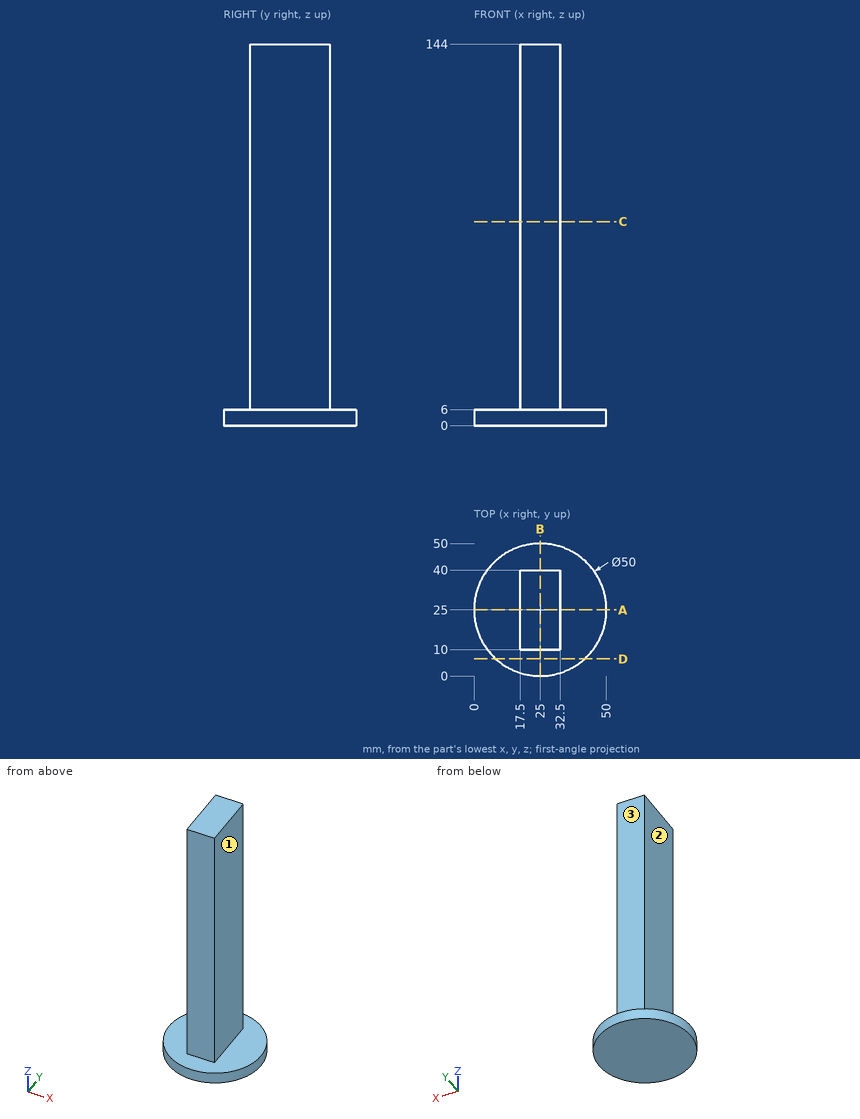
Print and shaded views of the part. All mm, measured from the part's lowest x, y and z. A direction names the side the tool comes from. Round coordinates to 2 decimals unless told otherwise and drop trailing zeros. Write each loop counter-clockwise with the first axis right and the second up, starting at its lowest first coordinate (ties: lowest second). Pieces come first, ordered by that corner, then holes.
(1) Slice it at C-C, the plane z = 77. Write the cut outline in (x, y).
(2) Slice it at D-D, the plane y = 6.5. Write the cut outline in (x, z).
(3) 3-axis set-ups, long thin cutter, end or side, ignore diameter. For the marked faces 1, 2 and 3: which of +Z, -Z, +X, -X, +Y, -Y reach the whole face in a straight line?
(4) Drop flat-ended pins along their axis: P1, Ø8, axis at x = 28.5, y = 23.5, coming from the -Z side; P2, Ø12, axis at x = 13, z = 18, coming from the -Y side; P3, Ø9, axis at y = 29, z = 60.5, coming from the -X side; P4, Ø24, axis at y = 29, z = 66.5, coming from the +X side. Give the stop position or say it passes through.
(5) Probe line 1 along Z through (x, y) = (34.5, 35); line 2 along Y through (x, z) = (21.5, 106); line 3 along X through (y, z) = (21, 31.5). List the from-to ranges inside material, lowest first.
(6) Slice it at B-B, the plane x = 25. Write the cut outline in (y, z), and give its area (3 significant figures).
(7) Slice it at A-A, the plane y = 25. Write the cut outline in (x, z), and give its area (3 significant figures).
From the geometry:
1. outline: (17.5, 10) - (32.5, 10) - (32.5, 40) - (17.5, 40) - close
2. outline: (8.18, 0) - (41.82, 0) - (41.82, 6) - (8.18, 6) - close
3. face 1: +Z, +X, +Y, -Y
3. face 2: +Z, -X, +Y, -Y
3. face 3: +Z, +X, -X, +Y
4. P1: stops at z = 0
4. P2: stops at y = 10
4. P3: stops at x = 17.5
4. P4: stops at x = 32.5
5. line 1: z = 0 to 6
5. line 2: y = 10 to 40
5. line 3: x = 17.5 to 32.5
6. outline: (0, 0) - (50, 0) - (50, 6) - (40, 6) - (40, 144) - (10, 144) - (10, 6) - (0, 6) - close
6. area: 4,440 mm2
7. outline: (0, 0) - (50, 0) - (50, 6) - (32.5, 6) - (32.5, 144) - (17.5, 144) - (17.5, 6) - (0, 6) - close
7. area: 2,370 mm2
